Work out the finished part from the listing and answer in its coordinate system (mm). Coordinates: 2 decimals unless noted, no trailing zeros. Loops run counter-clockwise (first coordinate to the right, second up) from the corner with the lowest first, then second, coordinate; pieces in that order, holes last. Notation, with made-up numbers: (79, 54) - (94, 54) arc R18 cw to (94, 81) - close; hole circle Ø1 at (-5.5, 76.5). An arc over 180 degrees is marked (long way). Write each question's results on one line, items separated by ' | '. Start each with the question number.
1. Each of these flat-tipped pins is pushed along its axis until it touches: P1, Ø2, axis at x = -13.5, z = 57, coming from the -Y side; P2, Ø1, axis at x = 15.5, z = 84.5, coming from the +Y side; P3, Ø8, axis at y = 25, z = 87.5, coming from the +X side. Where does it stop, or does it pass through?
2. Determine the mould class of faces 1 (the conical face through (41.82, 13.17, 67.17)), 2 (the flat face through (-9, 29, 0)), 3 (the conical face through (38.244, -15.857, 64.656)) for opening direction Y: released by +Y, released by -Y, zero draft, split by the parting line, or undercut.
3. A cutting plane is placed at C-C on z = 101.5. Determine the outline of the cut face in (x, y).
4. A cutting plane is placed at B-B on y = 0. Determine the outline of the cut face in (x, z).
5. A cutting plane is placed at A-A on x = 0. Determine the outline of the cut face in (y, z), then the cut area to 3 significant figures.
6. A cutting plane is placed at D-D on z = 155. Determine the outline of the cut face in (x, y).
7. Find the intervals of material crossed by line 1 along Y through (x, z) = (-40.5, 132.5); line 2 along X through (y, z) = (21.5, 109); line 3 along X through (y, z) = (-1.5, 27), in increasing order. Write a range as [from, to].
from build123d import *

# Parameters (mm, degrees)
BOX_W           = 200
BOX_H           = 199
BOX_DEPTH       = 200
BOX_PITCH_ANGLE = -10


with BuildPart() as cube:
    # Box → Box (new body)
    with BuildSketch(Plane.XY):
        with Locations((100, 99.5)):
            Rectangle(BOX_W, BOX_H)
    extrude(amount=BOX_DEPTH)


with BuildPart() as cube_1:
    # Box pitch: moved
    add(cube.part.rotate(Axis((0, 0, 0), (0, 1, 0)), BOX_PITCH_ANGLE))


with BuildPart() as cube_2:
    # Box placement: moved
    add(cube_1.part.moved(Location((-95, -94, 142))))


with BuildPart() as side_shade_64mm_base:
    # Sketch → Revolution (revolve)
    with BuildSketch(Plane.XZ):
        Polygon((32, 0), (61.975587, 170), (59.975587, 170), (30, 0), align=None)
    revolve(axis=Axis((0, 0, 0), (0, 0, 1)))

    # Cut: cut Cube
    add(cube_2.part, mode=Mode.SUBTRACT)


solid = side_shade_64mm_base.part
Values:
1) P1: y = -40.2 | P2: y = 44.46 | P3: x = 42.68
2) face 1: split by the parting line | face 2: zero draft | face 3: undercut
3) outline: circle Ø99.79 at (0, 0); hole circle Ø95.79 at (0, 0)
4) outline: (-58.18, 148.49) - (-32, 0) - (-30, 0) - (-56.24, 148.83) - close; (30, 0) - (32, 0) - (61.92, 169.67) - (59.85, 169.3) - close
5) outline: (-59.99, 158.75) - (-32, 0) - (-30, 0) - (-57.99, 158.75) - close; (30, 0) - (32, 0) - (59.99, 158.75) - (57.99, 158.75) - close | area: 635 mm^2
6) outline: (-21.27, -55.39) arc R59.33 ccw (long way) to (-21.27, 55.39) - (-21.27, 53.24) arc R57.33 cw (long way) to (-21.27, -53.24) - close
7) line 1: [-37.75, -34.75], [34.75, 37.75] | line 2: [-46.49, -44.28], [44.28, 46.49] | line 3: [-36.73, -34.73], [34.73, 36.73]
